```python
from build123d import *

# Parameters (mm, degrees)
BOSS_EXTRUDE1_DEPTH = 203.2
BOSS_EXTRUDE2_DEPTH = 160.02
SKETCH5_R           = 61.468
CUT_EXTRUDE1_DEPTH  = 25.4


with BuildPart() as part:
    # Sketch1 → Boss-Extrude1 (new body)
    with BuildSketch(Plane(origin=(0, 0, 0), x_dir=(1, 0, 0), z_dir=(0, 1, 0))):
        Polygon((0, 80), (-80, 80), (-80, 0), (-80, -80), (0, -80), (80, -80), (80, 0), (80, 80), align=None)
    extrude(amount=BOSS_EXTRUDE1_DEPTH)

    # Sketch4 → Boss-Extrude2 (add)
    with BuildSketch(Plane(origin=(80, 0, 0), x_dir=(0, 0, -1), z_dir=(1, 0, 0))):
        Polygon((80, 203.2), (-135.526146906, 545.726146906), (-240.337405258, 479.776242441), (-80, 203.2), align=None)
    extrude(amount=-BOSS_EXTRUDE2_DEPTH)

    # Sketch5 → Cut-Extrude1 (cut)
    with BuildSketch(Plane(origin=(0, 16.401175936, -28.291437078), x_dir=(1, 0, 0), z_dir=(0, -0.5015382826017037, 0.8651354524494611))):
        with Locations(Location((0, 372.618160976, 0), (0, 0, 270))):
            Circle(SKETCH5_R)
    extrude(amount=-CUT_EXTRUDE1_DEPTH, mode=Mode.SUBTRACT)


solid = part.part
```
Geometry check sheet. Reference: the model listing, model coordinates, mm. A direction names the side the tool comes from. Round coordinates to 2 decimals unless told otherwise and drop trailing zeros. Order: outer loops, then holes, each group sorted by start corner. A loop starts at its lowest first (then second) coordinate and runs counter-clockwise, first axis right, second up. Notation, with made-up numbers: (70, 3.25) - (110, 3.25) arc R34 cw to (110, 33.25) - close; hole circle Ø7 at (-24.75, 28). An arc over 180 degrees is marked (long way). Use a Markdown table: item, result. Add a question column.
1) Section check A-A (x = 51). Record the cut outline in (y, z).
2) Mould release check, pull along X, two halves, no side actions. Record for faces 1 (the cylindrical face through (18.463, 294.324, 118.352)), 2 (the flat face through (1.11, 372.065, 26.254)), 3 (the flat face through (-80, 100, -1)): released by +X, released by -X, zero draft, split by the parting line, or undercut.
3) Set-up check for faces 4 (the flat face through (-1, 100, 80)), 5 (the flat face through (-80.02, 339, 82)), 6 (the flat face through (0.86, 352.25, 137.05)): record each of +Z, -Z, +X, -X, +Y, -Y from which the full face is reachable in a straight line by a thin tool's end or side.
4) Section check B-B (y = 72). Record the cut outline in (x, z).
5) Gauge pin test, flat ends, axial feed: P1, Ø1, axis at x = -63.5, z = -42.5, coming from the +Y side; P2, Ø1.5, axis at x = 5.5, z = 39, coming from the +Y side. Record the tip position at first contact, or that the pin passes through.
6) Section check D-D (x = -48). Record the cut outline in (y, z), then the cut area to 3 significant figures.
7) Thickness scan on line 1 along Z through (x, y) = (29.5, 36.5); line 2 along Y through (x, z) = (46, 126). Record the ranges inside material, lowest first.
Established:
| question | item | result |
|---|---|---|
| 1 | outline | (0, -80) - (203.2, -80) - (545.73, 135.53) - (479.78, 240.34) - (368.45, 175.8) - (381.19, 153.83) - (321.82, 119.41) - (309.08, 141.38) - (203.2, 80) - (0, 80) - close |
| 2 | face 1 | undercut |
| 2 | face 2 | zero draft |
| 2 | face 3 | released by -X |
| 3 | face 4 | +Z, +X, -X, -Y |
| 3 | face 5 | +Z, -Z, -X, +Y, -Y |
| 3 | face 6 | none |
| 4 | outline | (-80, -80) - (80, -80) - (80, 80) - (-80, 80) - close |
| 5 | P1 | y = 263.59 |
| 5 | P2 | y = 393.51 |
| 6 | outline | (0, -80) - (203.2, -80) - (545.73, 135.53) - (479.78, 240.34) - (371.98, 177.85) - (384.72, 155.87) - (318.29, 117.36) - (305.55, 139.33) - (203.2, 80) - (0, 80) - close |
| 6 | area | 77,700 mm2 |
| 7 | line 1 | -80 to 80 |
| 7 | line 2 | 282.55 to 310.53, 333.19 to 530.59 |
